```python
from build123d import *

# Parameters (mm, degrees)
SKETCH1_W          = 470
SKETCH1_H          = 50
CUT_EXTRUDE2_DEPTH = 20


with BuildPart() as part:
    # Sketch1 → Revolve1 (revolve)
    with BuildSketch(Plane(origin=(0, 0, 0), x_dir=(0, 0, -1), z_dir=(1, 0, 0))):
        with Locations((-265, 0)):
            Rectangle(SKETCH1_W, SKETCH1_H)
    revolve(axis=Axis((0, 285.555555556, 0), (0, -1, 0)))

    # Sketch3 → Cut-Extrude2 (cut)
    with BuildSketch(Plane(origin=(0, 25, 0), x_dir=(1, 0, 0), z_dir=(0, 1, 0))):
        with BuildLine():
            Line((-45.632403393, 112.890460705), (-70, 171.719042916))
            ThreePointArc((-70, 171.719042916), (0, 185.438479556), (70, 171.719042916))
            Line((70, 171.719042916), (45.632403393, 112.890460705))
            ThreePointArc((45.632403393, 112.890460705), (0, 120), (-45.632403393, 112.890460705))
        make_face()
        with BuildLine():
            Line((112.092592177, 47.558628415), (170.921174388, 71.926225022))
            ThreePointArc((170.921174388, 71.926225022), (131.124806387, 131.124806387), (71.926225022, 170.921174388))
            Line((71.926225022, 170.921174388), (47.558628415, 112.092592177))
            ThreePointArc((47.558628415, 112.092592177), (84.852813742, 84.852813742), (112.092592177, 47.558628415))
        make_face()
        with BuildLine():
            Line((112.890460705, -45.632403393), (171.719042916, -70))
            ThreePointArc((171.719042916, -70), (185.438479556, 0), (171.719042916, 70))
            Line((171.719042916, 70), (112.890460705, 45.632403393))
            ThreePointArc((112.890460705, 45.632403393), (120, 0), (112.890460705, -45.632403393))
        make_face()
        with BuildLine():
            Line((47.558628415, -112.092592177), (71.926225022, -170.921174388))
            ThreePointArc((71.926225022, -170.921174388), (131.124806387, -131.124806387), (170.921174388, -71.926225022))
            Line((170.921174388, -71.926225022), (112.092592177, -47.558628415))
            ThreePointArc((112.092592177, -47.558628415), (84.852813742, -84.852813742), (47.558628415, -112.092592177))
        make_face()
        with BuildLine():
            Line((-45.632403393, -112.890460705), (-70, -171.719042916))
            ThreePointArc((-70, -171.719042916), (0, -185.438479556), (70, -171.719042916))
            Line((70, -171.719042916), (45.632403393, -112.890460705))
            ThreePointArc((45.632403393, -112.890460705), (0, -120), (-45.632403393, -112.890460705))
        make_face()
        with BuildLine():
            Line((-112.092592177, -47.558628415), (-170.921174388, -71.926225022))
            ThreePointArc((-170.921174388, -71.926225022), (-131.124806387, -131.124806387), (-71.926225022, -170.921174388))
            Line((-71.926225022, -170.921174388), (-47.558628415, -112.092592177))
            ThreePointArc((-47.558628415, -112.092592177), (-84.852813742, -84.852813742), (-112.092592177, -47.558628415))
        make_face()
        with BuildLine():
            Line((-112.890460705, 45.632403393), (-171.719042916, 70))
            ThreePointArc((-171.719042916, 70), (-185.438479556, 0), (-171.719042916, -70))
            Line((-171.719042916, -70), (-112.890460705, -45.632403393))
            ThreePointArc((-112.890460705, -45.632403393), (-120, 0), (-112.890460705, 45.632403393))
        make_face()
        with BuildLine():
            Line((-47.558628415, 112.092592177), (-71.926225022, 170.921174388))
            ThreePointArc((-71.926225022, 170.921174388), (-131.124806387, 131.124806387), (-170.921174388, 71.926225022))
            Line((-170.921174388, 71.926225022), (-112.092592177, 47.558628415))
            ThreePointArc((-112.092592177, 47.558628415), (-84.852813742, 84.852813742), (-47.558628415, 112.092592177))
        make_face()
    extrude(amount=-CUT_EXTRUDE2_DEPTH, mode=Mode.SUBTRACT)


solid = part.part
```
The model under review builds one solid part; all positions refer to its coordinate system, in mm. A direction names the side the tool comes from. Round coordinates to 2 decimals unless told otherwise and drop trailing zeros. Loops run counter-clockwise (first coordinate to the right, second up) from the corner with the lowest first, then second, coordinate; pieces in that order, holes last. Notation, with made-up numbers: (81, 72.5) -> (97, 72.5) arc R17 cw to (97, 85.5) -> close; hole circle Ø11 at (77, 17.5). An arc over 180 degrees is marked (long way). Answer as a JSON object with one key per item and string values. Group by question number.
1) We need section C-C on y = -6.5. Write out the cut boundary in (x, z).
2) Mouldability with a two-part tool opening along X and no side actions: class faces 1 (the face through (104, 25, -7)), 2 (the face through (-110, 5, 108)), 3 (the face through (141.919, 15.14, 59.913)) as released by +X, released by -X, zero draft, split by the parting line, or undercut.
3) For faces 4 (the face through (-57.646, 15.14, -141.893)), 5 (the face through (104, -25, -7)), list the 3-axis set-ups (+Z, -Z, +X, -X, +Y, -Y) from which the entire face can be reached by the end or side of a thin tool; tool diameter is ignored.
4) We need section B-B on x = 0. Write out the cut boundary in (y, z), then the cut area to 3 significant figures.
5) We need section A-A on z = 0. Write out the cut boundary in (x, y), then the cut area to 3 significant figures.
6) We need section D-D on x = -145.5. Write out the cut boundary in (y, z).
7) For line 1 (Z direction, x = 0, y = 8); line 2 (Z direction, x = 0, y = -5), list the stretches that pass through material, from the lowest coordinate up. Write a range as [from, to].
8) For pin 1 Ø12 at (y, z) = (-19, -202.5) entering from -X; pin 2 Ø1.5 at (y, z) = (-0.5, 346) entering from +X; pin 3 Ø3 at (y, z) = (17, 214) entering from -X, all flat-tipped, find the tip position at first contact; note any pin that passes through.
Result set:
{
 "1": {"outline": "circle Ø1000 at (0, 0); hole circle Ø60 at (0, 0)"},
 "2": {"face 1": "zero draft", "face 2": "undercut", "face 3": "undercut"},
 "3": {"face 4": "+Y", "face 5": "+Z, -Z, +X, -X, -Y"},
 "4": {"outline": "(-25, -500) -> (25, -500) -> (25, -185.44) -> (5, -185.44) -> (5, -120) -> (25, -120) -> (25, -30) -> (-25, -30) -> close; (-25, 30) -> (25, 30) -> (25, 120) -> (5, 120) -> (5, 185.44) -> (25, 185.44) -> (25, 500) -> (-25, 500) -> close", "area": "44,400 mm²"},
 "5": {"outline": "(-500, -25) -> (-30, -25) -> (-30, 25) -> (-120, 25) -> (-120, 5) -> (-185.44, 5) -> (-185.44, 25) -> (-500, 25) -> close; (30, -25) -> (500, -25) -> (500, 25) -> (185.44, 25) -> (185.44, 5) -> (120, 5) -> (120, 25) -> (30, 25) -> close", "area": "44,400 mm²"},
 "6": {"outline": "(-25, -478.36) -> (25, -478.36) -> (25, -114.97) -> (5, -114.97) -> (5, -61.4) -> (25, -61.4) -> (25, -59.14) -> (5, -59.14) -> (5, 59.14) -> (25, 59.14) -> (25, 61.4) -> (5, 61.4) -> (5, 114.97) -> (25, 114.97) -> (25, 478.36) -> (-25, 478.36) -> close"},
 "7": {"line 1": "[-500, -185.44], [-120, -30], [30, 120], [185.44, 500]", "line 2": "[-500, -30], [30, 500]"},
 "8": {"pin 1": "x = -459.77", "pin 2": "x = 361.67", "pin 3": "x = -452.6"}
}
